Build history of the part. All positions in model axes, mm. A direction names the side the tool comes from. Round coordinates to 2 decimals unless told otherwise and drop trailing zeros. Loops run counter-clockwise (first coordinate to the right, second up) from the corner with the lowest first, then second, coordinate; pieces in that order, holes last. Notation, with made-up numbers: (17.25, -38) - (57.25, -38) arc R26 cw to (57.25, -22) - close; hole circle Ø10 at (42.5, 19.25). An arc over 180 degrees is marked (long way). Put each result on its own line as item: value. Start each with the question number.
from build123d import *

# Parameters (mm, degrees)
SKETCH_1_W                 = 305.5
SKETCH_1_H                 = 1221.15
EXTRUDE_1_DEPTH            = 4.75
CUT_EXTRUDE_2_DEPTH        = 4.75
SPLIT_START                = 205.025
SPLIT_BODIES_2_OUTLINE_W   = 305.5
SPLIT_BODIES_2_OUTLINE_H   = 4.75
SPLIT_BODIES_2_DEPTH       = 405.55
SPLIT_START_2              = -610.575
SPLIT_BODIES_2_2_OUTLINE_W = 305.5
SPLIT_BODIES_2_2_OUTLINE_H = 4.75
SPLIT_BODIES_2_2_DEPTH     = 414.8


# Read off the part's stored shape, not the designer's step: 分割2
with BuildPart() as part:
    # 草圖1 → 填料-伸長1 (new body)
    with BuildSketch(Plane.XY):
        Rectangle(SKETCH_1_W, SKETCH_1_H)
    extrude(amount=EXTRUDE_1_DEPTH)

    # 草圖2 → 除料-伸長2 (cut)
    with BuildSketch(Plane.XY.offset(4.75)):
        Polygon((100.025, 354.412698413), (100.025, 304.423280423), (-83.25542328, 382.984126984), (-99.975, 390.137566138), (-99.975, 440.126984127), (83.30542328, 361.566137566), align=None)
        Polygon((57.189021164, 380.021164021), (57.189021164, 440.126984127), (100.025, 440.126984127), (100.025, 361.566137566), align=None)
        Polygon((50.035582011, 106.53968254), (57.189021164, 106.53968254), (57.189021164, 120.846560847), (100.025, 120.846560847), (100.025, 84.994708995), (71.453571429, 56.55026455), (50.035582011, 56.55026455), align=None)
        Polygon((-71.403571429, 56.55026455), (-99.975, 84.994708995), (-99.975, 120.846560847), (-57.096693122, 120.846560847), (-57.096693122, 106.53968254), (-21.414153439, 106.53968254), (-21.414153439, 120.846560847), (21.464153439, 120.846560847), (21.464153439, 85.121693122), (-7.107275132, 56.55026455), align=None)
        Polygon((-21.414153439, 142.264550265), (-57.096693122, 142.264550265), (-57.096693122, 127.830687831), (-99.975, 128), (-99.975, 163.682539683), (-71.403571429, 192.423280423), (71.453571429, 192.253968254), (100.025, 163.682539683), (100.025, 127.830687831), (57.189021164, 127.830687831), (57.189021164, 142.264550265), (21.464153439, 142.264550265), (21.464153439, 128), (-21.414153439, 128), align=None)
        Polygon((21.591137566, -141.164021164), (57.189021164, -141.164021164), (57.189021164, -127.026455026), (100.025, -127.026455026), (100.025, -162.878306878), (71.453571429, -191.322751323), (7.157275132, -191.322751323), (0.046164021, -184.042328042), (-6.980291005, -191.44973545), (-71.276587302, -191.44973545), (-99.848015873, -163.047619048), (-99.975, -127.026455026), (-57.096693122, -127.026455026), (-56.969708995, -141.333333333), (-21.24484127, -141.333333333), (-21.414153439, -127.026455026), (21.29484127, -126.899470899), (21.29484127, -127.153439153), (21.591137566, -127.153439153), align=None)
        Polygon((50.035582011, -55.44973545), (71.453571429, -55.44973545), (100.025, -84.19047619), (100.025, -120.042328042), (57.189021164, -120.042328042), (57.189021164, -105.608465608), (50.035582011, -105.608465608), align=None)
        Polygon((-49.985582011, -105.608465608), (-57.096693122, -105.608465608), (-57.096693122, -120.042328042), (-99.975, -119.873015873), (-99.975, -84.19047619), (-71.403571429, -55.44973545), (-49.985582011, -55.44973545), align=None)
        Polygon((50.035582011, -389.206349206), (57.189021164, -389.206349206), (57.189021164, -374.899470899), (100.025, -374.899470899), (100.025, -410.751322751), (71.453571429, -439.195767196), (50.035582011, -439.195767196), align=None)
        Polygon((-71.403571429, -439.195767196), (-99.975, -410.751322751), (-99.975, -374.899470899), (-57.096693122, -374.899470899), (-57.096693122, -389.206349206), (-21.414153439, -389.206349206), (-21.414153439, -374.899470899), (21.464153439, -374.899470899), (21.464153439, -410.624338624), (-7.107275132, -439.195767196), align=None)
        Polygon((-21.414153439, -353.481481481), (-57.096693122, -353.481481481), (-57.096693122, -367.915343915), (-99.975, -367.746031746), (-99.975, -332.063492063), (-71.403571429, -303.322751323), (71.453571429, -303.492063492), (100.025, -332.063492063), (100.025, -367.915343915), (57.189021164, -367.915343915), (57.189021164, -353.481481481), (21.464153439, -353.481481481), (21.464153439, -367.746031746), (-21.414153439, -367.746031746), align=None)
    extrude(amount=-CUT_EXTRUDE_2_DEPTH, mode=Mode.SUBTRACT)

    # Split Bodies 2 outline → Split Bodies 2 (cut)
    with BuildSketch(Plane(origin=(0, 0, 0), x_dir=(1, 0, 0), z_dir=(0, 1, 0)).offset(SPLIT_START)):
        with Locations((0, -2.375)):
            Rectangle(SPLIT_BODIES_2_OUTLINE_W, SPLIT_BODIES_2_OUTLINE_H)
    extrude(amount=SPLIT_BODIES_2_DEPTH, mode=Mode.SUBTRACT)

    # Split Bodies 2 2 outline → Split Bodies 2 2 (cut)
    with BuildSketch(Plane(origin=(0, 0, 0), x_dir=(1, 0, 0), z_dir=(0, 1, 0)).offset(SPLIT_START_2)):
        with Locations((0, -2.375)):
            Rectangle(SPLIT_BODIES_2_2_OUTLINE_W, SPLIT_BODIES_2_2_OUTLINE_H)
    extrude(amount=SPLIT_BODIES_2_2_DEPTH, mode=Mode.SUBTRACT)


solid = part.part
1) Which spindle directions (+Z, -Z, +X, -X, +Y, -Y) get a long thin tool onto all of the face, cutting with end or side? Do faces 3 (the face through (-2, 7, 4.75)), 4 (the face through (85.94, 70.97, 2.41)). Say none if no direction does.
2) Slice it at A-A, the plane y = 135. Write the cut outline in (x, z) (3 decimals).
3) Slice it at B-B, the plane x = 84. Write the cut outline in (y, z) (3 decimals), and give its area (3 significant figures).
4) Pull direction Y, two halves, no side cores. Call faces 1 (the face through (7.38, 71.04, 2.41)), 2 (the face through (-2, 7, 0)): pulls with the +Y half, pulls with the -Y half, needs draft (parallel to the pull), parting line crosses it, or undercut.
5) Drill centre lines: line 1 (X direction, y = 130.5, z = 1.9) (3 decimals); line 2 (Y direction, x = 26, z = 3.2) (3 decimals); line 3 (Y direction, x = 61, z = 3.6) (3 decimals). Where is each one in solid material? Low to high. Write a range as [from, to].
6) Slice it at D-D, the plane z = 3.6. State how many separate pieces and enclosed holes the cut face has, and give its area (3 significant figures).
7) Slice it at C-C, the plane y = -69.5. Write the cut outline in (x, z).
Taken from the geometry:
1. face 3: +Z, +X, -X, +Y, -Y
1. face 4: +Z, -Z
2. outline: (-152.75, 0) - (-99.975, 0) - (-99.975, 4.75) - (-152.75, 4.75) - close; (-57.097, 0) - (-21.414, 0) - (-21.414, 4.75) - (-57.097, 4.75) - close; (21.464, 0) - (57.189, 0) - (57.189, 4.75) - (21.464, 4.75) - close; (100.025, 0) - (152.75, 0) - (152.75, 4.75) - (100.025, 4.75) - close
3. outline: (-195.775, 0) - (-178.832, 0) - (-178.832, 4.75) - (-195.775, 4.75) - close; (-127.026, 0) - (-120.042, 0) - (-120.042, 4.75) - (-127.026, 4.75) - close; (-68.071, 0) - (69.041, 0) - (69.041, 4.75) - (-68.071, 4.75) - close; (120.847, 0) - (127.831, 0) - (127.831, 4.75) - (120.847, 4.75) - close; (179.708, 0) - (205.025, 0) - (205.025, 4.75) - (179.708, 4.75) - close
3. area: 918 mm2
4. face 1: undercut
4. face 2: needs draft
5. line 1: x = [-152.75, -99.975], [-57.097, -21.414], [21.464, 57.189], [100.025, 152.75]
5. line 2: y = [-195.775, -191.323], [-141.164, 142.265], [192.308, 205.025]
5. line 3: y = [-195.775, -191.323], [-127.026, -120.042], [-55.45, 56.55], [120.847, 127.831], [192.266, 205.025]
6. separate pieces: 1
6. enclosed holes: 6
6. area: 85,800 mm2
7. outline: (-152.75, 0) - (-85.37, 0) - (-85.37, 4.75) - (-152.75, 4.75) - close; (-49.99, 0) - (50.04, 0) - (50.04, 4.75) - (-49.99, 4.75) - close; (85.42, 0) - (152.75, 0) - (152.75, 4.75) - (85.42, 4.75) - close
